from build123d import *

# Parameters (mm, degrees)
F0_W         = 655
F0_H         = 30
F1_DEPTH     = 580
F3_DEPTH     = 13.5
F5_DEPTH     = 5
F6_R         = 51.5
F7_DEPTH     = 67
F9_DEPTH     = 47
F11_DEPTH    = 11
F13_DEPTH    = 210
F14_R        = 52.5
F15_DEPTH    = 8
F16_R        = 50
F17_DEPTH    = 13.5
F18_W        = 170
F18_H        = 120
F19_DEPTH    = 30
F20_SIZE     = 15
F21_T1_DEPTH = 68.5752448195
F22_W        = 655
F22_H        = 10
F23_DEPTH    = 71.7
F24_R        = 25
F25_DEPTH    = 42
F26_R        = 40
F27_DEPTH    = 50


# Not quite as in the source:
# - a fillet or chamfer that OpenCascade refuses, or shapes differently, is made with other operations: its cross-section is extruded or revolved along the edge and cut away or added


with BuildPart() as f1:
    # F0 (on Front) → F1 (new body)
    with BuildSketch(Plane.XZ):
        with Locations((35.6008394094, 15)):
            Rectangle(F0_W, F0_H)
    extrude(amount=F1_DEPTH)

    # F2 (on face) → F3 (join)
    with BuildSketch(Plane.XY.offset(30)):
        Polygon((-422.0060110092, -580), (233.1008394094, -580), (233.1008394094, -453), (-25.8483879637, 20), (-422.0060110092, 20), align=None)
    extrude(amount=F3_DEPTH)

    # F4 (on face) → F5 (cut)
    with BuildSketch(Plane.XY.offset(30)):
        with BuildLine():
            Line((315.5072791576, -218), (223.5072791576, -218))
            ThreePointArc((223.5072791576, -218), (217.8504249081, -220.3431457505), (215.5072791576, -226))
            Line((215.5072791576, -226), (215.5072791576, -353))
            ThreePointArc((215.5072791576, -353), (217.8504249081, -358.6568542495), (223.5072791576, -361))
            Line((223.5072791576, -361), (315.5072791576, -361))
            ThreePointArc((315.5072791576, -361), (321.1641334071, -358.6568542495), (323.5072791576, -353))
            Line((323.5072791576, -353), (323.5072791576, -226))
            ThreePointArc((323.5072791576, -226), (321.1641334071, -220.3431457505), (315.5072791576, -218))
        make_face()
    extrude(amount=-F5_DEPTH, mode=Mode.SUBTRACT)

    # F6 (on face) → F7 (join)
    with BuildSketch(Plane.XY.offset(25)):
        with Locations((269.5072791576, -289.5)):
            Circle(F6_R)
    extrude(amount=F7_DEPTH)

    # F8 (on face) → F9 (join)
    with BuildSketch(Plane.XY.offset(92)):
        with BuildLine():
            Line((331.5072791576, -219.5), (207.5072791576, -219.5))
            ThreePointArc((207.5072791576, -219.5), (201.8504249081, -221.8431457505), (199.5072791576, -227.5))
            Line((199.5072791576, -227.5), (199.5072791576, -351.5))
            ThreePointArc((199.5072791576, -351.5), (201.8504249081, -357.1568542495), (207.5072791576, -359.5))
            Line((207.5072791576, -359.5), (331.5072791576, -359.5))
            ThreePointArc((331.5072791576, -359.5), (337.1641334071, -357.1568542495), (339.5072791576, -351.5))
            Line((339.5072791576, -351.5), (339.5072791576, -227.5))
            ThreePointArc((339.5072791576, -227.5), (337.1641334071, -221.8431457505), (331.5072791576, -219.5))
        make_face()
    extrude(amount=F9_DEPTH)

    # F10 (on face) → F11 (join)
    with BuildSketch(Plane.XY.offset(139)):
        with BuildLine():
            Line((329.8072791576, -216.7), (209.2072791576, -216.7))
            ThreePointArc((209.2072791576, -216.7), (200.3684443928, -220.3611652352), (196.7072791576, -229.2))
            Line((196.7072791576, -229.2), (196.7072791576, -349.8))
            ThreePointArc((196.7072791576, -349.8), (200.3684443928, -358.6388347648), (209.2072791576, -362.3))
            Line((209.2072791576, -362.3), (329.8072791576, -362.3))
            ThreePointArc((329.8072791576, -362.3), (338.6461139225, -358.6388347648), (342.3072791576, -349.8))
            Line((342.3072791576, -349.8), (342.3072791576, -229.2))
            ThreePointArc((342.3072791576, -229.2), (338.6461139225, -220.3611652352), (329.8072791576, -216.7))
        make_face()
    extrude(amount=F11_DEPTH)

    # F12 (on face) → F13 (join)
    with BuildSketch(Plane.XY.offset(150)):
        with BuildLine():
            ThreePointArc((221.6497197978, -359.5550261631), (222.4537040204, -361.4960157773), (224.3946936347, -362.3))
            Line((224.3946936347, -362.3), (314.5623053207, -362.3))
            ThreePointArc((314.5623053207, -362.3), (316.503294935, -361.4960157773), (317.3072791576, -359.5550261631))
            Line((317.3072791576, -359.5550261631), (317.3072791576, -349.8))
            ThreePointArc((317.3072791576, -349.8), (320.7925325094, -341.1406499743), (329.3047740164, -337.3101045407))
            ThreePointArc((329.3047740164, -337.3101045407), (329.8072791576, -337.3), (330.3097842989, -337.3101045407))
            Line((330.3097842989, -337.3101045407), (339.5623053207, -337.3101045407))
            ThreePointArc((339.5623053207, -337.3101045407), (341.503294935, -336.5061203181), (342.3072791576, -334.5651307038))
            Line((342.3072791576, -334.5651307038), (342.3072791576, -244.4433875239))
            ThreePointArc((342.3072791576, -244.4433875239), (341.503294935, -242.5023979096), (339.5623053207, -241.698413687))
            Line((339.5623053207, -241.698413687), (330.006415567, -241.698413687))
            ThreePointArc((330.006415567, -241.698413687), (321.7732212328, -238.7762160199), (317.4644895357, -231.1762450125))
            ThreePointArc((317.4644895357, -231.1762450125), (317.3072791576, -229.2), (317.4644895357, -227.2237549875))
            Line((317.4644895357, -227.2237549875), (317.4644895357, -219.4449738369))
            ThreePointArc((317.4644895357, -219.4449738369), (316.6605053131, -217.5039842227), (314.7195156988, -216.7))
            Line((314.7195156988, -216.7), (224.4374317064, -216.7))
            ThreePointArc((224.4374317064, -216.7), (222.4949663799, -217.5054610577), (221.6924610453, -219.4491493681))
            Line((221.6924610453, -219.4491493681), (221.7072646957, -229.18098556))
            ThreePointArc((221.7072646957, -229.18098556), (218.1514308097, -237.9322477762), (209.4879256393, -241.696849105))
            ThreePointArc((209.4879256393, -241.696849105), (209.2072791576, -241.7), (208.926632676, -241.696849105))
            Line((208.926632676, -241.696849105), (199.4522529946, -241.696849105))
            ThreePointArc((199.4522529946, -241.696849105), (197.5112633803, -242.5008333276), (196.7072791576, -244.4418229419))
            Line((196.7072791576, -244.4418229419), (196.7072791576, -334.5586429094))
            ThreePointArc((196.7072791576, -334.5586429094), (197.5112633803, -336.4996325237), (199.4522529946, -337.3036167464))
            Line((199.4522529946, -337.3036167464), (208.906603954, -337.3036167464))
            ThreePointArc((208.906603954, -337.3036167464), (209.2072791576, -337.3), (209.5079543613, -337.3036167464))
            ThreePointArc((209.5079543613, -337.3036167464), (217.722501739, -340.6489899798), (221.6497197978, -348.6018051423))
            ThreePointArc((221.6497197978, -348.6018051423), (221.7072791576, -349.8), (221.6497197978, -350.9981948577))
            Line((221.6497197978, -350.9981948577), (221.6497197978, -359.5550261631))
        make_face()
        with BuildLine():
            Line((221.6497197978, -348.6018051423), (221.6497197978, -350.9981948577))
            ThreePointArc((221.6497197978, -350.9981948577), (221.7072791576, -349.8), (221.6497197978, -348.6018051423))
        make_face()
        with BuildLine():
            ThreePointArc((330.3097842989, -337.3101045407), (329.8072791576, -337.3), (329.3047740164, -337.3101045407))
            Line((329.3047740164, -337.3101045407), (330.3097842989, -337.3101045407))
        make_face()
        with BuildLine():
            Line((208.906603954, -337.3036167464), (209.5079543613, -337.3036167464))
            ThreePointArc((209.5079543613, -337.3036167464), (209.2072791576, -337.3), (208.906603954, -337.3036167464))
        make_face()
        with BuildLine():
            Line((209.4879256393, -241.696849105), (208.926632676, -241.696849105))
            ThreePointArc((208.926632676, -241.696849105), (209.2072791576, -241.7), (209.4879256393, -241.696849105))
        make_face()
        with BuildLine():
            ThreePointArc((317.4644895357, -227.2237549875), (317.3072791576, -229.2), (317.4644895357, -231.1762450125))
            Line((317.4644895357, -231.1762450125), (317.4644895357, -227.2237549875))
        make_face()
    extrude(amount=F13_DEPTH)

    # F14 (on face) → F15 (join)
    with BuildSketch(Plane.XY.offset(360)):
        with Locations((269.5072791576, -289.5)):
            Circle(F14_R)
    extrude(amount=F15_DEPTH)

    # F16 (on face) → F17 (cut)
    with BuildSketch(Plane.XY.offset(43.5)):
        with Locations((-113.8991605906, -340.5)):
            Circle(F16_R)
    extrude(amount=-F17_DEPTH, mode=Mode.SUBTRACT)

    # F18 (on face) → F19 (join)
    with BuildSketch(Plane.XY.offset(43.5)):
        with Locations((-113.8991605906, -90.5)):
            Rectangle(F18_W, F18_H)
        Polygon((-424.8670357638, -421.8878406783), (-339.8670357638, -569.1121593217), (-235.9439873097, -509.1121593217), (-320.9439873097, -361.8878406783), align=None)
        Polygon((112.0687145825, -569.1121593217), (197.0687145825, -421.8878406783), (93.1456661284, -361.8878406783), (8.1456661284, -509.1121593217), align=None)
    extrude(amount=F19_DEPTH)

    # F20
    f20_edges = [f1.edges().sort_by_distance(p)[0] for p in [
        (-198.899161, -30.5, 58.5),
    ]]
    chamfer(f20_edges, length=F20_SIZE)

    # F21: chamfer of 15 on 11 edges, made by hand

    # F21_s2 → F21_t1 (cut)
    with BuildSketch(Plane.XY.offset(43.5)):
        Polygon((-43.8991605906, -30.5), (-28.8991605906, -45.5), (-28.8991605906, -30.5), align=None)
        Polygon((106.1360471852, -369.3878406783), (85.6456661284, -374.8782217351), (93.1456661284, -361.8878406783), align=None)
        Polygon((15.6456661284, -496.1217782649), (21.1360471852, -516.6121593217), (8.1456661284, -509.1121593217), align=None)
        Polygon((119.5687145825, -556.1217782649), (99.0783335258, -561.6121593217), (112.0687145825, -569.1121593217), align=None)
        Polygon((189.5687145825, -434.8782217351), (184.0783335258, -414.3878406783), (197.0687145825, -421.8878406783), align=None)
        Polygon((-28.8991605906, -135.5), (-43.8991605906, -150.5), (-28.8991605906, -150.5), align=None)
        Polygon((-198.8991605906, -135.5), (-183.8991605906, -150.5), (-198.8991605906, -150.5), align=None)
        Polygon((-248.9343683664, -516.6121593217), (-243.4439873097, -496.1217782649), (-235.9439873097, -509.1121593217), align=None)
        Polygon((-347.3670357638, -556.1217782649), (-326.876654707, -561.6121593217), (-339.8670357638, -569.1121593217), align=None)
        Polygon((-417.3670357638, -434.8782217351), (-411.876654707, -414.3878406783), (-424.8670357638, -421.8878406783), align=None)
        Polygon((-313.4439873097, -374.8782217351), (-333.9343683664, -369.3878406783), (-320.9439873097, -361.8878406783), align=None)
    extrude(amount=F21_T1_DEPTH, mode=Mode.SUBTRACT)

    # F22 (on face) → F23 (join)
    with BuildSketch(Plane(origin=(0, 0, 0), x_dir=(1, 0, 0), z_dir=(0, 0, -1))):
        with Locations((35.6008394094, 105)):
            Rectangle(F22_W, F22_H)
        with Locations((35.6008394094, 447)):
            Rectangle(F22_W, F22_H)
    extrude(amount=F23_DEPTH)

    # F24 (on face) → F25 (join)
    with BuildSketch(Plane(origin=(0, 0, 0), x_dir=(1, 0, 0), z_dir=(0, 0, -1))):
        with Locations((269.5072791576, 289.5)):
            Circle(F24_R)
    extrude(amount=F25_DEPTH)

    # F26 (on face) → F27 (join)
    with BuildSketch(Plane(origin=(0, 0, -42), x_dir=(1, 0, 0), z_dir=(0, 0, -1))):
        with Locations((269.5072791576, 289.5)):
            Circle(F26_R)
    extrude(amount=F27_DEPTH)


solid = f1.part
Input: part model. Units: mm. Frame: model coordinates. A direction names the side the tool comes from. Coordinates: 2 decimals unless noted, no trailing zeros. Loops run counter-clockwise (first coordinate to the right, second up) from the corner with the lowest first, then second, coordinate; pieces in that order, holes last. Notation, with made-up numbers: (-11.75, -27) - (-0.75, -27) arc R15 cw to (-0.75, -7) - close; hole circle Ø2 at (0.25, 55). An arc over 180 degrees is marked (long way). Answer in a Markdown table with one row per item. Add a question column.
Item 1: Line query: line 1 along Y through (x, z) = (86, -60); line 2 along Y through (x, z) = (249, -19); line 3 along Z through (x, y) = (-236, -487). Output: solid intervals per line, ascending. Write a range as [from, to].
Item 2: Mould query, pull axis X, two halves, no side actions, for faces 1 (the flat face through (18.35, -506.22, 58.29)), 2 (the flat face through (-115, -30.5, 58)), 3 (the flat face through (-172, -276, 43.5)), 4 (the flat face through (199.507, -289, 115)). Classes: released by +X, released by -X, zero draft, split by the parting line, or undercut.
Item 3: Section query B-B on x = -218. Return the cut outline in (y, z), then the cut area to 3 significant figures.
Item 4: Contact query for flat-ended pins moving along their axis: P1, Ø23.5, axis at y = -313.5, z = 119.5, coming from the -X side; P2, Ø1, axis at y = -296.5, z = 184.5, coming from the +X side; P3, Ø2.5, axis at x = 261.5, z = 26.5, coming from the +Y side. Output: stop coordinate, or through.
Item 5: Section query A-A on z = -58.5. Return the cut outline in (x, y), then the cut area to 3 significant figures.
Item 6: Section query D-D on x = -123.5. Return the cut outline in (y, z), then the cut area to 3 significant figures.
Item 7: Section query C-C on y = -84. Return the cut outline in (x, z).
Item 8: Access query for faces 5 (the flat face through (207, -230, 150)), 6 (the flat face through (-277.954, -436.349, 58.29)), 7 (the flat face through (31, -110, -35)), 8 (the flat face through (328, -351, 150)), 9 (the flat face through (-288.451, -539.427, 58.29)). Directions: +Z, -Z, +X, -X, +Y, -Y. A direction counts if a zero-diameter tool reaches every point of the face in a straight line with its end or side. Return the directions, or none.
Recorded:
| question | item | result |
|---|---|---|
| 1 | line 1 | [-452, -442], [-110, -100] |
| 1 | line 2 | [-452, -442], [-303.8, -275.2], [-110, -100] |
| 1 | line 3 | [0, 43.5] |
| 2 | face 1 | undercut |
| 2 | face 2 | zero draft |
| 2 | face 3 | undercut |
| 2 | face 4 | released by -X |
| 3 | outline | (-580, 0) - (-452, 0) - (-452, -71.7) - (-442, -71.7) - (-442, 0) - (-110, 0) - (-110, -71.7) - (-100, -71.7) - (-100, 0) - (0, 0) - (0, 30) - (20, 30) - (20, 43.5) - (-580, 43.5) - close |
| 3 | area | 26,900 mm^2 |
| 4 | P1 | x = 199.51 |
| 4 | P2 | x = 342.31 |
| 4 | P3 | y = 0 |
| 5 | outline | (-291.9, -452) - (363.1, -452) - (363.1, -442) - (-291.9, -442) - close; (-291.9, -110) - (363.1, -110) - (363.1, -100) - (-291.9, -100) - close; circle Ø80 at (269.51, -289.5) |
| 5 | area | 18,100 mm^2 |
| 6 | outline | (-580, 0) - (-452, 0) - (-452, -71.7) - (-442, -71.7) - (-442, 0) - (-110, 0) - (-110, -71.7) - (-100, -71.7) - (-100, 0) - (0, 0) - (0, 30) - (20, 30) - (20, 43.5) - (-30.5, 43.5) - (-30.5, 73.5) - (-150.5, 73.5) - (-150.5, 43.5) - (-291.43, 43.5) - (-291.43, 30) - (-389.57, 30) - (-389.57, 43.5) - (-580, 43.5) - close |
| 6 | area | 29,200 mm^2 |
| 7 | outline | (-422.01, 30) - (-291.9, 30) - (-291.9, 0) - (363.1, 0) - (363.1, 30) - (31.09, 30) - (31.09, 43.5) - (-28.9, 43.5) - (-28.9, 73.5) - (-198.9, 73.5) - (-198.9, 43.5) - (-422.01, 43.5) - close |
| 8 | face 5 | +Z, -X, +Y |
| 8 | face 6 | +Z, +Y |
| 8 | face 7 | -Z, +X, -X |
| 8 | face 8 | +Z, +X, -Y |
| 8 | face 9 | +Z, -Y |
